Work out the finished part from the listing and answer in its coordinate system (mm). Face numbers are marked on the shaded views. A direction names the side the tool comes from. Round coordinates to 2 decimals unless told otherwise and drop trailing zeros. Write each loop counter-clockwise with the first axis right and the second up, starting at its lowest first coordinate (ties: lowest second). Pieces come first, ordered by that corner, then holes. Notation, with made-up numbers: M 48,-19.75 L 73,-19.75 A17 ccw 73,5.25 Z; hole C -39.5,44 d9. An arc over 180 degrees is marked long. One line per item, written item: value. Start each with the question number.
Q1. Find section B-B (x = 9). Write down the section's boundary in (y, z).
Q2. A tool of negligible diameter and unlimited length cuts with its end or side. For the marked faces 1 and 2, from which of +Z, -Z, +X, -X, +Y, -Y can it reach the whole face along a straight path? Write none if from no direction.
Q3. Given pin 1 Ø20 at (y, z) = (-45.5, 19) entering from +X, flat-ended and moving along its own axis, determine where the tip first touches the part or whether it passes through.
Q4. Find section C-C (z = 12). Write down the section's boundary in (x, y), and give its area (3 significant figures).
Q5. Consider probe 1 along Y at (x, z) = (-38, 25); probe 2 along X at (y, z) = (-67, 44.5); probe 3 along Y at (x, z) = (-4, 29.5). Determine where each line is inside the solid, lowest interval first.
Q6. Find section D-D (y = -39). Write down the section's boundary in (x, z).
Q7. Find section A-A (z = 25). Write down the section's boundary in (x, y).
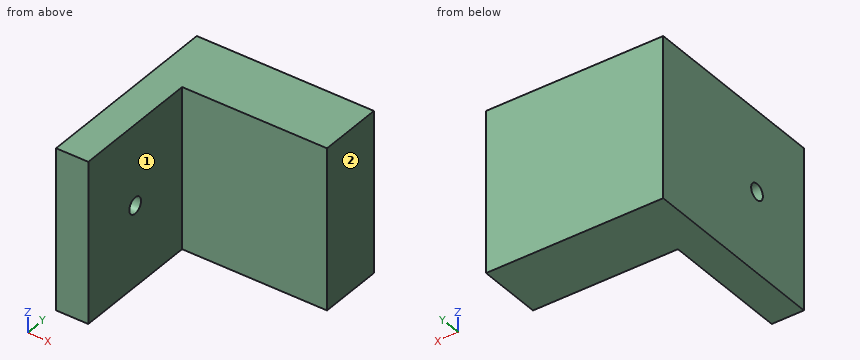
from build123d import *

# Parameters (mm, degrees)
SALIENTE_EXTRUIR1_DEPTH                        = 50
PERFORADOR_PARA_ROSCAR_PARA_MACHO_DE_ROS_D     = 5
PERFORADOR_PARA_ROSCAR_PARA_MACHO_DE_ROS_DEPTH = 11
PERFORADOR_PARA_ROSCAR_PARA_MACHO_DE_ROS_TIP   = 1.502151548


with BuildPart() as part:
    # Croquis1 → Saliente-Extruir1 (new body)
    with BuildSketch(Plane.XY):
        Polygon((-42.31300039, -15.146269262), (12.68699961, -15.146269262), (12.68699961, -35.146269262), (-32.31300039, -35.146269262), (-32.31300039, -75.146269262), (-42.31300039, -75.146269262), align=None)
    extrude(amount=SALIENTE_EXTRUIR1_DEPTH)

    # Perforador para roscar para macho de roscar para M6x1.01
    with Locations(Plane(origin=(-32.31300039, -55.146269262, 25), x_dir=(0, 0, 1), z_dir=(1, 0, 0))):
        with Locations((0, 0)):
            Hole(PERFORADOR_PARA_ROSCAR_PARA_MACHO_DE_ROS_D / 2, depth=PERFORADOR_PARA_ROSCAR_PARA_MACHO_DE_ROS_DEPTH)
            with Locations((0, 0, -(PERFORADOR_PARA_ROSCAR_PARA_MACHO_DE_ROS_DEPTH + PERFORADOR_PARA_ROSCAR_PARA_MACHO_DE_ROS_TIP / 2))):  # 118° drill point
                Cone(0, PERFORADOR_PARA_ROSCAR_PARA_MACHO_DE_ROS_D / 2, PERFORADOR_PARA_ROSCAR_PARA_MACHO_DE_ROS_TIP, mode=Mode.SUBTRACT)


solid = part.part
The answers:
1. outline: M -35.15,0 L -15.15,0 L -15.15,50 L -35.15,50 Z
2. face 1: +Z, -Z, +X, -Y
2. face 2: +Z, -Z, +X, +Y, -Y
3. pin 1: x = -32.31
4. outline: M -42.31,-75.15 L -32.31,-75.15 L -32.31,-35.15 L 12.69,-35.15 L 12.69,-15.15 L -42.31,-15.15 Z
4. area: 1,500 mm2
5. probe 1: -75.15 to -57.65, -52.65 to -15.15
5. probe 2: -42.31 to -32.31
5. probe 3: -35.15 to -15.15
6. outline: M -42.31,0 L -32.31,0 L -32.31,50 L -42.31,50 Z
7. outline: M -42.31,-75.15 L -32.31,-75.15 L -32.31,-57.65 L -42.31,-57.65 Z; M -42.31,-52.65 L -32.31,-52.65 L -32.31,-35.15 L 12.69,-35.15 L 12.69,-15.15 L -42.31,-15.15 Z
